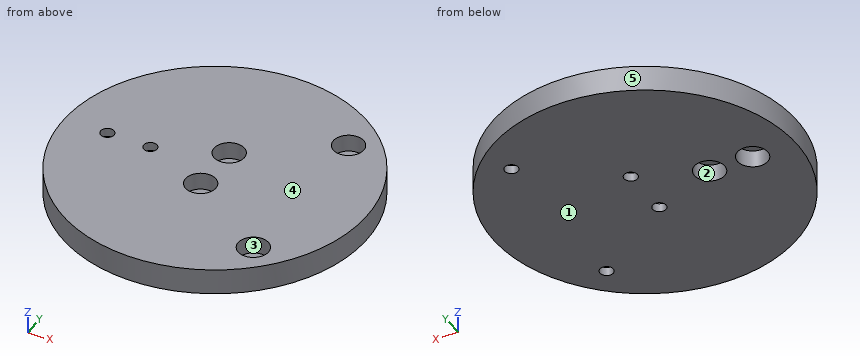
from build123d import *

# Parameters (mm, degrees)
F0_R     = 35
F1_DEPTH = 6
F2_R     = 1.55
F3_DEPTH = 6
F4_R     = 3.5
F4_R_2   = 1.55
F5_DEPTH = 4
F6_R     = 3.5
F7_DEPTH = 4


# Not quite as in the source:
# - a feature names something its author has since deleted; it is built from what else it names


with BuildPart() as f1:
    # F0 (on Top) → F1 (new body)
    with BuildSketch(Plane.XY):
        Circle(F0_R)
    extrude(amount=F1_DEPTH)

    # F2 (on face) → F3 (cut, through all)
    with BuildSketch(Plane.XY.offset(6)):
        with Locations((0, 6)):
            Circle(F2_R)
        with Locations((0, -6)):
            Circle(F2_R)
        with Locations((20, 20)):
            Circle(F2_R)
        with Locations((20, -20)):
            Circle(F2_R)
        with Locations((-15, 0)):
            Circle(F2_R)
        with Locations((-25, 0)):
            Circle(F2_R)
    extrude(amount=-F3_DEPTH, mode=Mode.SUBTRACT)

    # F4 (on face) → F5 (cut)
    with BuildSketch(Plane.XY.offset(6)):
        with Locations((0, -6)):
            Circle(F4_R)
        with Locations((0, 6)):
            Circle(F4_R)
        with Locations((20, -20)):
            Circle(F4_R)
        with Locations((20, 20)):
            Circle(F4_R)
        with Locations((20, 20)):
            Circle(F4_R_2)
        with Locations((20, -20)):
            Circle(F4_R_2)
    extrude(amount=-F5_DEPTH, mode=Mode.SUBTRACT)

    # F6 (on face) → F7 (cut)
    with BuildSketch(Plane(origin=(0, 0, 0), x_dir=(1, 0, 0), z_dir=(0, 0, -1))):
        with Locations((-25, 0)):
            Circle(F6_R)
        with Locations((-15, 0)):
            Circle(F6_R)
    extrude(amount=-F7_DEPTH, mode=Mode.SUBTRACT)


solid = f1.part
For this review, take the finished solid that the model builds, in its own axes (mm). Face numbers are marked on the shaded views. A direction names the side the tool comes from. Round coordinates to 2 decimals unless told otherwise and drop trailing zeros. Loops run counter-clockwise (first coordinate to the right, second up) from the corner with the lowest first, then second, coordinate; pieces in that order, holes last. Notation, with made-up numbers: (-5, 88) - (8, 88) arc R23 ccw to (8, 118) - close; hole circle Ø2 at (-24, 6). An arc over 180 degrees is marked (long way). One line per item, written item: value. Start each with the question number.
Item 1: Take a section at C-C (y = 0). Give the boundary of the cut face in (x, z), plus the area to 3 significant figures.
Item 2: Take a section at B-B (x = 0). Give the boundary of the cut face in (y, z), plus the area to 3 significant figures.
Item 3: For L1, parallel to Y at x = 20, z = 0.9; L2, parallel to Y at x = 1.5, z = 4.2; L3, parallel to X at y = -2.5, z = 1.75, list the stretches that pass through material, from the lowest coordinate up.
Item 4: Take a section at A-A (z = 2.95). Give the boundary of the cut face in (x, y).
Item 5: Clearance check with flat-ended pins moving along their axes: pin 1 Ø2 at (y, z) = (13.5, 1) entering from +X; pin 2 Ø1 at (x, z) = (-11.5, 5.5) entering from +Y; pin 3 Ø4 at (x, y) = (0, 6) entering from +Z; pin 4 Ø3 at (x, y) = (0, 6) entering from -Z. State where each tip first meets the part, or that it passes through.
Item 6: Take a section at D-D (x = -15). Give the boundary of the cut face in (y, z).
Item 7: The part is to be moulded in two halves that separate along X. For the marked faces 3, 4 and 5, say which applies: +X half, -X half, draft (parallel to the pull), parting line (faces both ways), or undercut.
Item 8: For the marked faces 1 and 2, list the 3-axis set-ups (+Z, -Z, +X, -X, +Y, -Y) from which the entire face can be reached by the end or side of a thin tool; tool diameter is ignored.
Answer below:
1. outline: (-35, 0) - (-28.5, 0) - (-28.5, 4) - (-26.55, 4) - (-26.55, 6) - (-35, 6) - close; (-23.45, 4) - (-21.5, 4) - (-21.5, 0) - (-18.5, 0) - (-18.5, 4) - (-16.55, 4) - (-16.55, 6) - (-23.45, 6) - close; (-13.45, 4) - (-11.5, 4) - (-11.5, 0) - (35, 0) - (35, 6) - (-13.45, 6) - close
1. area: 352 mm2
2. outline: (-35, 0) - (-7.55, 0) - (-7.55, 2) - (-9.5, 2) - (-9.5, 6) - (-35, 6) - close; (-4.45, 0) - (4.45, 0) - (4.45, 2) - (2.5, 2) - (2.5, 6) - (-2.5, 6) - (-2.5, 2) - (-4.45, 2) - close; (7.55, 0) - (35, 0) - (35, 6) - (9.5, 6) - (9.5, 2) - (7.55, 2) - close
2. area: 352 mm2
3. L1: y = -28.72 to -21.55, -18.45 to 18.45, 21.55 to 28.72
3. L2: y = -34.97 to -9.16, -2.84 to 2.84, 9.16 to 34.97
3. L3: x = -34.91 to -27.45, -22.55 to -17.45, -12.55 to 34.91
4. outline: circle Ø70 at (0, 0); hole circle Ø7 at (-25, 0); hole circle Ø7 at (-15, 0); hole circle Ø7 at (0, -6); hole circle Ø7 at (0, 6); hole circle Ø7 at (20, -20); hole circle Ø7 at (20, 20)
5. pin 1: stops at x = 32.69
5. pin 2: stops at y = 33.23
5. pin 3: stops at z = 2
5. pin 4: passes through
6. outline: (-31.62, 0) - (-3.5, 0) - (-3.5, 4) - (-1.55, 4) - (-1.55, 6) - (-31.62, 6) - close; (1.55, 4) - (3.5, 4) - (3.5, 0) - (31.62, 0) - (31.62, 6) - (1.55, 6) - close
7. face 3: undercut
7. face 4: draft
7. face 5: parting line
8. face 1: -Z, +X, -X, +Y, -Y
8. face 2: -Z
